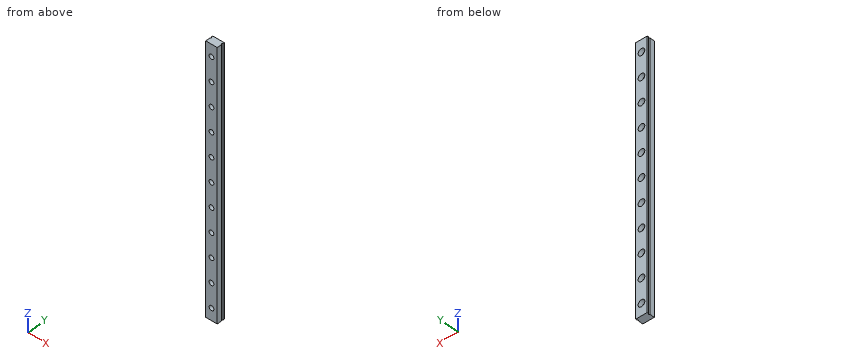
from build123d import *

# Parameters (mm, degrees)
BOSS_EXTRUDE1_DEPTH = 275
SKETCH2_R           = 2.5
CUT_EXTRUDE1_DEPTH  = 9
SKETCH2_3_R         = 3.5
SKETCH2_3_R_2       = 2.5
CUT_EXTRUDE2_DEPTH  = 4.5


with BuildPart() as part:
    # Sketch1 → Boss-Extrude1 (new body)
    with BuildSketch(Plane.XY):
        Polygon((6, -3), (6, 1.666666667), (5.166666667, 2.5), (6, 3.333333333), (6, 5), (-6, 5), (-6, 3.333333333), (-5.166666667, 2.5), (-6, 1.666666667), (-6, -3), align=None)
    extrude(amount=BOSS_EXTRUDE1_DEPTH)

    # Sketch2 → Cut-Extrude1 (cut, through all)
    with BuildSketch(Plane(origin=(0, 5, 0), x_dir=(1, 0, 0), z_dir=(0, 1, 0))):
        with Locations((0, -12.5)):
            Circle(SKETCH2_R)
        with Locations((0, -262.5)):
            Circle(SKETCH2_R)
        with Locations((0, -137.5)):
            Circle(SKETCH2_R)
        with Locations((0, -37.5)):
            Circle(SKETCH2_R)
        with Locations((0, -62.5)):
            Circle(SKETCH2_R)
        with Locations((0, -87.5)):
            Circle(SKETCH2_R)
        with Locations((0, -112.5)):
            Circle(SKETCH2_R)
        with Locations((0, -162.5)):
            Circle(SKETCH2_R)
        with Locations((0, -187.5)):
            Circle(SKETCH2_R)
        with Locations((0, -212.5)):
            Circle(SKETCH2_R)
        with Locations((0, -237.5)):
            Circle(SKETCH2_R)
    extrude(amount=-CUT_EXTRUDE1_DEPTH, mode=Mode.SUBTRACT)

    # Sketch2<3> → Cut-Extrude2 (cut)
    with BuildSketch(Plane(origin=(0, 5, 0), x_dir=(1, 0, 0), z_dir=(0, 1, 0))):
        with Locations((0, -12.5)):
            Circle(SKETCH2_3_R)
        with Locations((0, -12.5)):
            Circle(SKETCH2_3_R_2, mode=Mode.SUBTRACT)
        with Locations((0, -262.5)):
            Circle(SKETCH2_3_R)
        with Locations((0, -262.5)):
            Circle(SKETCH2_3_R_2, mode=Mode.SUBTRACT)
        with Locations((0, -137.5)):
            Circle(SKETCH2_3_R)
        with Locations((0, -137.5)):
            Circle(SKETCH2_3_R_2, mode=Mode.SUBTRACT)
        with Locations((0, -37.5)):
            Circle(SKETCH2_3_R)
        with Locations((0, -37.5)):
            Circle(SKETCH2_3_R_2, mode=Mode.SUBTRACT)
        with Locations((0, -62.5)):
            Circle(SKETCH2_3_R)
        with Locations((0, -62.5)):
            Circle(SKETCH2_3_R_2, mode=Mode.SUBTRACT)
        with Locations((0, -87.5)):
            Circle(SKETCH2_3_R)
        with Locations((0, -87.5)):
            Circle(SKETCH2_3_R_2, mode=Mode.SUBTRACT)
        with Locations((0, -112.5)):
            Circle(SKETCH2_3_R)
        with Locations((0, -112.5)):
            Circle(SKETCH2_3_R_2, mode=Mode.SUBTRACT)
        with Locations((0, -162.5)):
            Circle(SKETCH2_3_R)
        with Locations((0, -162.5)):
            Circle(SKETCH2_3_R_2, mode=Mode.SUBTRACT)
        with Locations((0, -187.5)):
            Circle(SKETCH2_3_R)
        with Locations((0, -187.5)):
            Circle(SKETCH2_3_R_2, mode=Mode.SUBTRACT)
        with Locations((0, -212.5)):
            Circle(SKETCH2_3_R)
        with Locations((0, -212.5)):
            Circle(SKETCH2_3_R_2, mode=Mode.SUBTRACT)
        with Locations((0, -237.5)):
            Circle(SKETCH2_3_R)
        with Locations((0, -237.5)):
            Circle(SKETCH2_3_R_2, mode=Mode.SUBTRACT)
    extrude(amount=-CUT_EXTRUDE2_DEPTH, mode=Mode.SUBTRACT)


solid = part.part
The listing builds one solid part. Answer for the finished solid, in the listing's coordinates (mm). Coordinates: 2 decimals unless noted, no trailing zeros. Loops run counter-clockwise (first coordinate to the right, second up) from the corner with the lowest first, then second, coordinate; pieces in that order, holes last.
1) Find section A-A on z = 262.5. Write down the section's boundary in (x, y), then the cut area to 3 significant figures.
2) A flat-ended cylindrical pin translates along its axis: pin 1 Ø3.5 at (x, z) = (1, 138) entering from +Y. Find the tip coordinate at first contact, or state that the pin passes through.
3) Find the intervals of material crossed by L1, parallel to X at y = -0.25, z = 237.5; L2, parallel to X at y = 3, z = 211; L3, parallel to Y at x = 5.25, z = 191.5, in increasing order.
4) Find section B-B on y = -1. Give the number of separate pieces and of enclosed holes in the cut face, then the cut area to 3 significant figures.
Values:
1. outline: (-6, -3) - (-2.5, -3) - (-2.5, 0.5) - (-3.5, 0.5) - (-3.5, 5) - (-6, 5) - (-6, 3.33) - (-5.17, 2.5) - (-6, 1.67) - close; (2.5, -3) - (6, -3) - (6, 1.67) - (5.17, 2.5) - (6, 3.33) - (6, 5) - (3.5, 5) - (3.5, 0.5) - (2.5, 0.5) - close
1. area: 45.6 mm2
2. pin 1: stops at y = 0.5
3. L1: x = -6 to -2.5, 2.5 to 6
3. L2: x = -5.67 to -3.16, 3.16 to 5.67
3. L3: y = -3 to 2.42, 2.58 to 5
4. separate pieces: 1
4. enclosed holes: 11
4. area: 3,080 mm2
